The model under review builds one solid part; all positions refer to its coordinate system, in mm. Face numbers are marked on the shaded views. A direction names the side the tool comes from. Coordinates: 2 decimals unless noted, no trailing zeros. Order: outer loops, then holes, each group sorted by start corner. A loop starts at its lowest first (then second) coordinate and runs counter-clockwise, first axis right, second up.
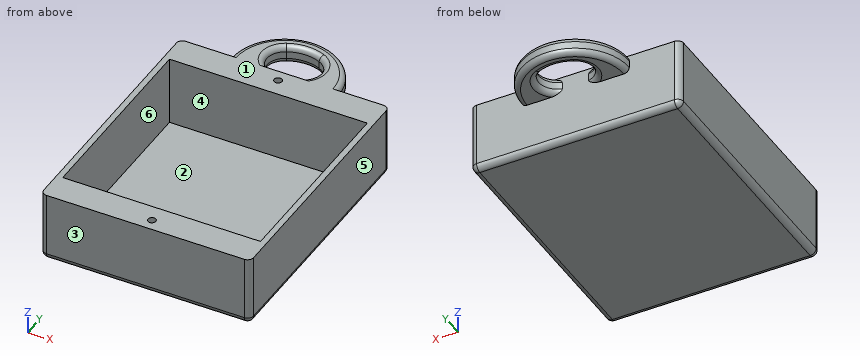
from build123d import *

# Parameters (mm, degrees)
SKETCH_W        = 35.1
SKETCH_H        = 43.1
PAD_DEPTH       = 11.72
SKETCH002_W     = 33.1
SKETCH002_H     = 33.1
POCKET_DEPTH    = 11.6
SKETCH006_R     = 0.65
POCKET004_DEPTH = 5
PAD002_DEPTH    = 3
FILLET_R        = 1
FILLET002_R     = 0.9


with BuildPart() as part:
    # Sketch → Pad (new body)
    with BuildSketch(Plane.XY):
        Rectangle(SKETCH_W, SKETCH_H)
    extrude(amount=PAD_DEPTH)

    # Sketch002 (on Face6 of Pad) → Pocket (cut)
    with BuildSketch(Plane.XY.offset(11.72)):
        Rectangle(SKETCH002_W, SKETCH002_H)
    extrude(amount=-POCKET_DEPTH, mode=Mode.SUBTRACT)

    # Sketch006 (on Face5 of Pocket) → Pocket004 (cut)
    with BuildSketch(Plane.XY.offset(11.72)):
        with Locations((0, 19.55)):
            Circle(SKETCH006_R)
        with Locations((0, -19.55)):
            Circle(SKETCH006_R)
    extrude(amount=-POCKET004_DEPTH, mode=Mode.SUBTRACT)

    # Sketch008 (on Face5 of Pocket004) → Pad002 (join)
    with BuildSketch(Plane.XY.offset(11.72)):
        with BuildLine():
            ThreePointArc((9, 21.55), (0, 30.55), (-9, 21.55))
            Line((-2.210805, 21.55), (-9, 21.55))
            ThreePointArc((-2.834383, 27.399468), (-4.579363, 24.255474), (-2.210805, 21.55))
            ThreePointArc((2.58169, 27.515306), (-0.138989, 28.048514), (-2.834383, 27.399468))
            ThreePointArc((2.210805, 21.55), (4.490762, 24.40243), (2.58169, 27.515306))
            Line((9, 21.55), (2.210805, 21.55))
        make_face()
    extrude(amount=-PAD002_DEPTH)

    # Fillet
    fillet_edges = [part.edges().sort_by_distance(p)[0] for p in [
        (-17.55, -21.55, 5.86),
        (-17.55, 0, 0),
        (0, -21.55, 0),
        (17.55, -21.55, 5.86),
        (17.55, 0, 0),
        (-17.55, 21.55, 5.86),
        (0, 21.55, 0),
        (17.55, 21.55, 5.86),
    ]]
    fillet(fillet_edges, radius=FILLET_R)

    # Fillet002
    fillet002_edges = [part.edges().sort_by_distance(p)[0] for p in [
        (0, 30.55, 11.72),
        (0, 30.55, 8.72),
        (-4.579363, 24.255474, 8.72),
        (-0.138989, 28.048514, 8.72),
        (4.490762, 24.40243, 8.72),
        (-4.579363, 24.255474, 11.72),
        (-0.138989, 28.048514, 11.72),
        (4.490762, 24.40243, 11.72),
    ]]
    fillet(fillet002_edges, radius=FILLET002_R)


solid = part.part
(1) Consider section B-B (y = -9.5). Give the boundary of the cut face in (x, z).
(2) Wall thickness on line 1 (Y direction, x = 0, z = 7.7); line 2 (Y direction, x = 0, z = 10.3); line 3 (Y direction, x = 0, z = 9.45): over which ranges is each line inside the solid? List them lowest first.
(3) Consider section C-C (x = -11.5). Give the boundary of the cut face in (y, z).
(4) Insertion check: pin 1 Ø1 at (x, y) = (0, -19.5) entering from +Z; pin 2 Ø9 at (x, y) = (0.5, 27.5) entering from -Z; pin 3 Ø16.5 at (x, y) = (-4, 1.5) entering from +Z. Each pin has a flat end and moves straight along its axis. Give the tip position at first contact, or say it passes through.
(5) Tool access review of the marked faces 1 and 2: name each direction out of +Z, -Z, +X, -X, +Y, -Y from which nothing blocks a thin tool from reaching the whole face with its end or side.
(6) Consider section A-A (z = 3). Give the boundary of the cut face in (x, y).
(7) The part is to be moulded in two halves that separate along Y. For the marked faces 3, 4, 5 and 6, say which applies: +Y half, -Y half, draft (parallel to the pull), parting line (faces both ways), or undercut.
Findings:
1. outline: (-17.55, 1) arc R1 ccw to (-16.55, 0) - (16.55, 0) arc R1 ccw to (17.55, 1) - (17.55, 11.72) - (16.55, 11.72) - (16.55, 0.12) - (-16.55, 0.12) - (-16.55, 11.72) - (-17.55, 11.72) - close
2. line 1: y = -21.55 to -20.2, -18.9 to -16.55, 16.55 to 18.9, 20.2 to 21.55
2. line 2: y = -21.55 to -20.2, -18.9 to -16.55, 16.55 to 18.9, 20.2 to 21.55, 28.05 to 30.55
2. line 3: y = -21.55 to -20.2, -18.9 to -16.55, 16.55 to 18.9, 20.2 to 21.55, 28.07 to 30.53
3. outline: (-21.55, 1) arc R1 ccw to (-20.55, 0) - (20.55, 0) arc R1 ccw to (21.55, 1) - (21.55, 11.72) - (16.55, 11.72) - (16.55, 0.12) - (-16.55, 0.12) - (-16.55, 11.72) - (-21.55, 11.72) - close
4. pin 1: stops at z = 6.72
4. pin 2: stops at z = 8.72
4. pin 3: stops at z = 0.12
5. face 1: +Z, +X, -X, +Y, -Y
5. face 2: +Z
6. outline: (-17.55, -20.55) arc R1 ccw to (-16.55, -21.55) - (16.55, -21.55) arc R1 ccw to (17.55, -20.55) - (17.55, 20.55) arc R1 ccw to (16.55, 21.55) - (-16.55, 21.55) arc R1 ccw to (-17.55, 20.55) - close; hole (-16.55, -16.55) - (16.55, -16.55) - (16.55, 16.55) - (-16.55, 16.55) - close
7. face 3: -Y half
7. face 4: undercut
7. face 5: draft
7. face 6: undercut
